Read the model definition and answer for the solid it produces. Units are mm, in the model's axes. Face numbers are marked on the shaded views. A direction names the side the tool comes from. Coordinates: 2 decimals unless noted, no trailing zeros. Order: outer loops, then holes, each group sorted by start corner. A loop starts at its lowest first (then second) coordinate and runs counter-clockwise, first axis right, second up. Notation, with made-up numbers: (-35.75, 13) - (-12.75, 13) arc R29 ccw to (-12.75, 40) - close; hole circle Ø6 at (-29.75, 20). An arc over 180 degrees is marked (long way). Use one line per item in the form item = value. Start each with the question number.
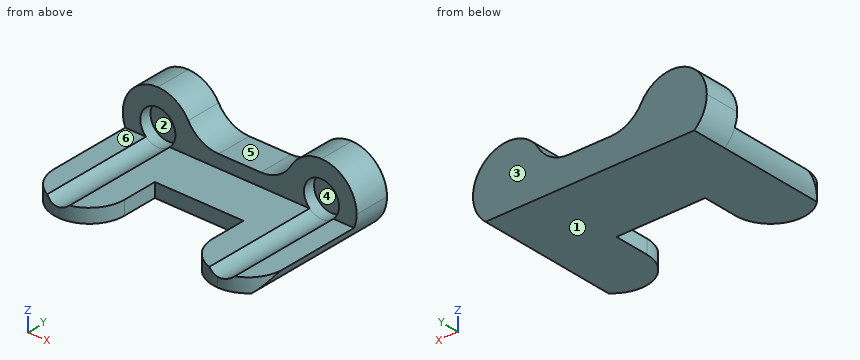
from build123d import *

# Parameters (mm, degrees)
F0_R      = 9.525
F1_DEPTH  = 25.4
F3_DEPTH  = 63.5
F4_DEPTH  = 46.228
F5_R      = 19.05
F6_R      = 9.525
F7_DEPTH  = 19.05
F8_DEPTH  = 6.35
F10_DEPTH = 25.4
F11_W     = 17.3040702939
F11_H     = 4.6345468581
F12_DEPTH = 12.7
F13_W     = 23.2714904292
F13_H     = 5.4139880085
F14_DEPTH = 12.7
F16_DEPTH = 25.4
F17_DEPTH = 25.4


with BuildPart() as f1:
    # F0 (on Front) → F1 (new body)
    with BuildSketch(Plane.XZ):
        with BuildLine():
            Line((-44.45, -19.05), (44.45, -19.05))
            ThreePointArc((44.45, -19.05), (30.9796158184, -13.4703841816), (25.4, 0))
            Line((25.4, 0), (-25.4, 0))
            ThreePointArc((-25.4, 0), (-30.9796158184, -13.4703841816), (-44.45, -19.05))
        make_face()
        with BuildLine():
            ThreePointArc((-63.5, 0), (-57.9203841816, -13.4703841816), (-44.45, -19.05))
            ThreePointArc((-44.45, -19.05), (-30.9796158184, -13.4703841816), (-25.4, 0))
            ThreePointArc((-25.4, 0), (-30.9796158184, 13.4703841816), (-44.45, 19.05))
            ThreePointArc((-44.45, 19.05), (-57.9203841816, 13.4703841816), (-63.5, 0))
        make_face()
        with Locations((-44.45, 0)):
            Circle(F0_R, mode=Mode.SUBTRACT)
        with BuildLine():
            ThreePointArc((25.4, 0), (30.9796158184, -13.4703841816), (44.45, -19.05))
            ThreePointArc((44.45, -19.05), (57.9203841816, -13.4703841816), (63.5, 0))
            ThreePointArc((63.5, 0), (57.9203841816, 13.4703841816), (44.45, 19.05))
            ThreePointArc((44.45, 19.05), (30.9796158184, 13.4703841816), (25.4, 0))
        make_face()
        with Locations((44.45, 0)):
            Circle(F0_R, mode=Mode.SUBTRACT)
    extrude(amount=F1_DEPTH)

    # F2 (on face) → F3 (join)
    with BuildSketch(Plane.XZ.offset(25.4)):
        with BuildLine():
            Line((-50.9257547823, -6.985), (-62.1732128859, -6.985))
            ThreePointArc((-62.1732128859, -6.985), (-59.9041022043, -11.1388161426), (-56.6809637805, -14.605))
            Line((-56.6809637805, -14.605), (56.6809637805, -14.605))
            ThreePointArc((56.6809637805, -14.605), (59.9041022043, -11.1388161426), (62.1732128859, -6.985))
            Line((62.1732128859, -6.985), (50.9257547823, -6.985))
            ThreePointArc((50.9257547823, -6.985), (44.45, -9.525), (37.9742452177, -6.985))
            Line((37.9742452177, -6.985), (-37.9742452177, -6.985))
            ThreePointArc((-37.9742452177, -6.985), (-44.45, -9.525), (-50.9257547823, -6.985))
        make_face()
    extrude(amount=F3_DEPTH)

    # F4 (cut): a face of the model
    f4_faces = [f1.faces().sort_by_distance(p)[0] for p in [
        (0, -25.4, -16.7601163622),
    ]]
    extrude(f4_faces, amount=-F4_DEPTH, mode=Mode.SUBTRACT)

    # F5
    f5_edges = [f1.edges().sort_by_distance(p)[0] for p in [
        (-25.4, -12.7, 0),
        (25.4, -12.7, 0),
    ]]
    fillet(f5_edges, radius=F5_R)

    # F6 (on face) → F7 (join)
    with BuildSketch(Plane(origin=(0, 0, 0), x_dir=(-1, 0, 0), z_dir=(0, 1, 0))):
        with Locations((-44.45, 0)):
            Circle(F6_R)
        with Locations((44.45, 0)):
            Circle(F6_R)
    extrude(amount=-F7_DEPTH)

    # F8 (cut): a face of the model
    f8_faces = [f1.faces().sort_by_distance(p)[0] for p in [
        (0, 0, -1.1785637601),
    ]]
    extrude(f8_faces, amount=-F8_DEPTH, mode=Mode.SUBTRACT)

    # F9 (on face) → F10 (cut)
    with BuildSketch(Plane.XY.offset(-6.985)):
        Polygon((24.0732128859, -69.85), (24.0732128859, -50.8), (-24.0732128859, -50.8), (-24.0732128859, -69.85), (-24.0732128859, -88.9), (24.0732128859, -88.9), align=None)
    extrude(amount=-F10_DEPTH, mode=Mode.SUBTRACT)

    # F11 (on face) → F12 (join)
    with BuildSketch(Plane.XZ.offset(88.9)):
        with Locations((-43.290130794, -9.3022734291)):
            Rectangle(F11_W, F11_H)
    extrude(amount=-F12_DEPTH)

    # F13 (on face) → F14 (join)
    with BuildSketch(Plane.XZ.offset(88.9)):
        with Locations((42.6594742664, -9.6919940042)):
            Rectangle(F13_W, F13_H)
    extrude(amount=-F14_DEPTH)

    # F15 (on face) → F16 (cut)
    with BuildSketch(Plane.XY.offset(-6.985)):
        with BuildLine():
            Line((62.1732128859, -88.9), (62.1732128859, -69.85))
            ThreePointArc((62.1732128859, -69.85), (56.5935970675, -83.3203841816), (43.1232128859, -88.9))
            Line((43.1232128859, -88.9), (50.9257547823, -88.9))
            Line((50.9257547823, -88.9), (54.295219481, -88.9))
            Line((54.295219481, -88.9), (62.1732128859, -88.9))
        make_face()
        with BuildLine():
            Line((37.9742452177, -88.9), (43.1232128859, -88.9))
            ThreePointArc((43.1232128859, -88.9), (29.6528287043, -83.3203841816), (24.0732128859, -69.85))
            Line((24.0732128859, -69.85), (24.0732128859, -88.9))
            Line((24.0732128859, -88.9), (31.0237290518, -88.9))
            Line((31.0237290518, -88.9), (37.9742452177, -88.9))
        make_face()
        with BuildLine():
            Line((-24.0732128859, -88.9), (-24.0732128859, -69.85))
            ThreePointArc((-24.0732128859, -69.85), (-29.6528287043, -83.3203841816), (-43.1232128859, -88.9))
            Line((-43.1232128859, -88.9), (-37.9742452177, -88.9))
            Line((-37.9742452177, -88.9), (-34.6380956471, -88.9))
            Line((-34.6380956471, -88.9), (-24.0732128859, -88.9))
        make_face()
        with BuildLine():
            Line((-50.9257547823, -88.9), (-43.1232128859, -88.9))
            ThreePointArc((-43.1232128859, -88.9), (-56.5935970675, -83.3203841816), (-62.1732128859, -69.85))
            Line((-62.1732128859, -69.85), (-62.1732128859, -88.9))
            Line((-62.1732128859, -88.9), (-51.942165941, -88.9))
            Line((-51.942165941, -88.9), (-50.9257547823, -88.9))
        make_face()
    extrude(amount=-F16_DEPTH, mode=Mode.SUBTRACT)

    # F17 (cut): faces of the model
    f17_faces = [f1.faces().sort_by_distance(p)[0] for p in [
        (44.45, -76.2, -8.0135872996),
        (-44.45, -76.2, -8.0135872996),
    ]]
    extrude(f17_faces, amount=-F17_DEPTH, mode=Mode.SUBTRACT)


solid = f1.part
Q1. A cutting plane is placed at A-A (y = -62). Give the vertices of the cut face in (x, z) (3 decimals), then the cut area to 3 significant figures.
Q2. For a pull along X with two mould halves and no side action, classify the marked faces 1 and 2 as +X half, -X half, draft (parallel to the pull), parting line (faces both ways), or undercut.
Q3. A cutting plane is placed at B-B (y = -44). Give the vertices of the cut face in (x, z) (3 decimals).
Q4. A cutting plane is placed at C-C (z = 14.5). Give the vertices of the cut face in (x, y).
Q5. Which of the six approach directions +Z, -Z, +X, -X, +Y, -Y give full straight-line access (tool end or side, diameter ignored) to the marked faces 3, 4, 5 and 6?
Q6. Given P1, Ø1.5, axis at x = -10, z = -4.5, coming from the -Y side; P2, Ø5, axis at x = 45, y = -56, coming from the +Z side; P3, Ø17, axis at x = 44.45, z = 0, coming from the -Y side; P4, Ø5, axis at x = 1.5, z = 2, coming from the +Y side, each flat-ended and moving along its own axis, determine where each tip first touches the part or whether it passes through.
Q7. Consider probe 1 along Z at (x, y) = (-44.45, -22.5) (3 decimals); probe 2 along X at (y, z) = (-46, -8.5); probe 3 along Y at (x, z) = (-45, 13). Determine where each line is inside the solid, lowest interval first.
Result sheet:
q1.outline = (-62.173, -6.985) arc R19.05 ccw to (-56.681, -14.605) - (-24.073, -14.605) - (-24.073, -6.985) - (-37.974, -6.985) arc R9.525 cw to (-50.926, -6.985) - close; (24.073, -14.605) - (56.681, -14.605) arc R19.05 ccw to (62.173, -6.985) - (50.926, -6.985) arc R9.525 cw to (37.974, -6.985) - (24.073, -6.985) - close
q1.area = 501 mm^2
q2.face_1 = draft
q2.face_2 = undercut
q3.outline = (-62.173, -6.985) arc R19.05 ccw to (-56.681, -14.605) - (56.681, -14.605) arc R19.05 ccw to (62.173, -6.985) - (50.926, -6.985) arc R9.525 cw to (37.974, -6.985) - (-37.974, -6.985) arc R9.525 cw to (-50.926, -6.985) - close
q4.outline = (-56.81, -25.4) - (-32.09, -25.4) - (-32.09, -6.35) - (-56.81, -6.35) - close; (32.09, -25.4) - (56.81, -25.4) - (56.81, -6.35) - (32.09, -6.35) - close
q5.face_3 = +Z, -Z, +X, -X, +Y
q5.face_4 = -Y
q5.face_5 = +Z, +Y, -Y
q5.face_6 = +Z, +X, -X, -Y
q6.P1 = -25.4
q6.P2 = -9.02
q6.P3 = -19.05
q6.P4 = -6.35
q7.probe_1 = -14.605 to -9.525, 9.525 to 19.05
q7.probe_2 = -61.5 to -48.75, -40.15 to 40.15, 48.75 to 61.5
q7.probe_3 = -25.4 to -6.35
